from build123d import *

# Parameters (mm, degrees)
SKETCH001_W     = 49
SKETCH001_H     = 49
PAD_DEPTH       = 1
SKETCH002_W     = 35
SKETCH002_H     = 35
PAD001_DEPTH    = 8
SKETCH003_W     = 25
SKETCH003_H     = 25
POCKET_DEPTH    = 10
SKETCH004_R     = 0.75
POCKET001_DEPTH = 2
SKETCH005_R     = 0.75
POCKET002_DEPTH = 10


with BuildPart() as part:
    # Sketch001 → Pad (new body, symmetric)
    with BuildSketch(Plane.XY):
        with Locations((24.5, 24.5)):
            Rectangle(SKETCH001_W, SKETCH001_H)
    extrude(amount=PAD_DEPTH, both=True)

    # Sketch002 (on Face6 of Pad) → Pad001 (join)
    with BuildSketch(Plane.XY.offset(1)):
        with Locations((24.5, 24.5)):
            Rectangle(SKETCH002_W, SKETCH002_H)
    extrude(amount=PAD001_DEPTH)

    # Sketch003 (on Face11 of Pad001) → Pocket (cut)
    with BuildSketch(Plane.XY.offset(9)):
        with Locations((24.5, 24.5)):
            Rectangle(SKETCH003_W, SKETCH003_H)
    extrude(amount=-POCKET_DEPTH, mode=Mode.SUBTRACT)

    # Sketch004 (on Face5 of Pocket) → Pocket001 (cut)
    with BuildSketch(Plane.XY.offset(1)):
        with Locations((3.5, 3.5)):
            Circle(SKETCH004_R)
        with Locations((3.5, 45.5)):
            Circle(SKETCH004_R)
        with Locations((45.5, 3.5)):
            Circle(SKETCH004_R)
        with Locations((45.5, 45.5)):
            Circle(SKETCH004_R)
    extrude(amount=-POCKET001_DEPTH, mode=Mode.SUBTRACT)

    # Sketch005 (on Face19 of Pocket001) → Pocket002 (cut)
    with BuildSketch(Plane.XY.offset(9)):
        with Locations((9.5, 39.5)):
            Circle(SKETCH005_R)
        with Locations((39.5, 39.5)):
            Circle(SKETCH005_R)
        with Locations((39.5, 9.5)):
            Circle(SKETCH005_R)
        with Locations((9.5, 9.5)):
            Circle(SKETCH005_R)
    extrude(amount=-POCKET002_DEPTH, mode=Mode.SUBTRACT)


solid = part.part
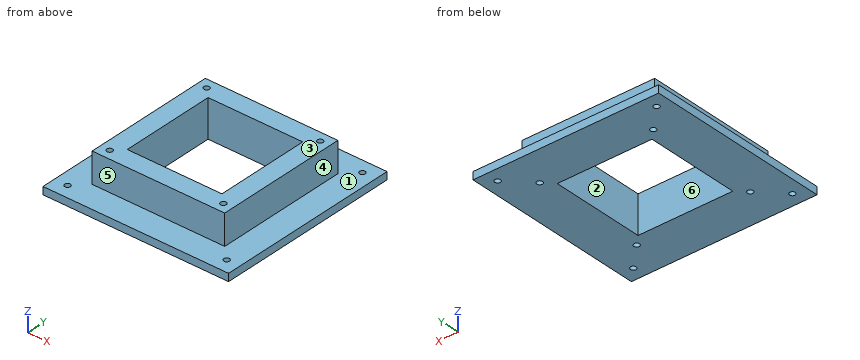
Check sheet for the modelled part. Datum: model origin and axes. Units: mm. Face numbers are marked on the shaded views. A direction names the side the tool comes from. Round coordinates to 2 decimals unless told otherwise and drop trailing zeros. Loops run counter-clockwise (first coordinate to the right, second up) from the corner with the lowest first, then second, coordinate; pieces in that order, holes last. Notation, with made-up numbers: (-36.75, 71) -> (-25.75, 71) arc R36 cw to (-25.75, 110) -> close; hole circle Ø5 at (-25.5, 53). An arc over 180 degrees is marked (long way). Put each result on its own line as item: value. Start each with the question number.
1. Draft check along X on the marked faces 4, 5 and 6. Enter one of: +X half, -X half, draft (parallel to the pull), parting line (faces both ways), or undercut.
2. Gauge pin test, flat ends, axial feed: pin 1 (0.9 mm diameter, centred on x = 39.5, y = 39.5, fed in from +Z); pin 2 (2.5 mm diameter, centred on x = 22, z = 4.5, fed in from +Y); pin 3 (4 mm diameter, centred on y = 17.5, z = 3.5, fed in from -X); pin 4 (4 mm diameter, centred on x = 22.5, z = 6, fed in from -Y). Record the tip position at first contact, or that the pin passes through.
3. Section check A-A (y = 24). Enter the section's corners in (x, z), plus the area to 3 significant figures.
4. Access from +Z, -Z, +X, -X, +Y, -Y to the whole of each face (thin tool, end or side, straight path). Record for the marked faces 1, 2 and 3.
5. Section check C-C (y = 9.5). Enter the section's corners in (x, z), plus the area to 3 significant figures.
6. Scan lines: probe 1 along Y at (x, z) = (39.5, 6.75); probe 2 along Y at (x, z) = (3.5, 0.3). Record each from-to range of solid material in increasing order.
Findings:
1. face 4: +X half
1. face 5: draft
1. face 6: undercut
2. pin 1: passes through
2. pin 2: stops at y = 42
2. pin 3: stops at x = 7
2. pin 4: stops at y = 7
3. outline: (0, -1) -> (12, -1) -> (12, 9) -> (7, 9) -> (7, 1) -> (0, 1) -> close; (37, -1) -> (49, -1) -> (49, 1) -> (42, 1) -> (42, 9) -> (37, 9) -> close
3. area: 128 mm^2
4. face 1: +Z
4. face 2: +Z, -Z
4. face 3: +Z, +X, -X, +Y, -Y
5. outline: (0, -1) -> (8.75, -1) -> (8.75, 9) -> (7, 9) -> (7, 1) -> (0, 1) -> close; (10.25, -1) -> (38.75, -1) -> (38.75, 9) -> (10.25, 9) -> close; (40.25, -1) -> (49, -1) -> (49, 1) -> (42, 1) -> (42, 9) -> (40.25, 9) -> close
5. area: 348 mm^2
6. probe 1: y = 7 to 8.75, 10.25 to 38.75, 40.25 to 42
6. probe 2: y = 0 to 2.75, 4.25 to 44.75, 46.25 to 49
